Input: part model. Units: mm. Frame: model coordinates. Face numbers are marked on the shaded views. A direction names the side the tool comes from. Coordinates: 2 decimals unless noted, no trailing zeros. Order: outer loops, then holes, each group sorted by start corner. A loop starts at its lowest first (then second) coordinate and runs counter-clockwise, first axis right, second up.
from build123d import *

# Parameters (mm, degrees)
F0_R     = 1.27
F1_DEPTH = 13.096875
F2_W     = 19.84375
F2_H     = 11.90625
F3_DEPTH = 30.1635
F5_DEPTH = 26.19475
F7_R     = 4.7625
F8_DEPTH = 22.226


with BuildPart() as f1:
    # F0 (on Top) → F1 (new body, symmetric)
    with BuildSketch(Plane.XY):
        Polygon((-15.08125, 0), (0, 0), (15.08125, 0), (15.08125, 26.19375), (7.14375, 26.19375), (7.14375, 7.9375), (0, 7.9375), (-7.14375, 7.9375), (-7.14375, 26.19375), (-15.08125, 26.19375), align=None)
        with Locations((-11.1125, 22.225)):
            Circle(F0_R, mode=Mode.SUBTRACT)
        with Locations((11.1125, 22.225)):
            Circle(F0_R, mode=Mode.SUBTRACT)
    extrude(amount=F1_DEPTH, both=True)

    # F2 (on face) → F3 (cut, through all)
    with BuildSketch(Plane(origin=(-15.08125, 0, 0), x_dir=(0, -1, 0), z_dir=(-1, 0, 0))):
        with Locations((-16.271875, 7.14375)):
            Rectangle(F2_W, F2_H)
    extrude(amount=-F3_DEPTH, mode=Mode.SUBTRACT)

    # F4 (on face) → F5 (cut, through all)
    with BuildSketch(Plane.XZ):
        with BuildLine():
            ThreePointArc((-2.54, 13.096875), (0, 10.556875), (2.54, 13.096875))
            Line((2.54, 13.096875), (-2.54, 13.096875))
        make_face()
    extrude(amount=-F5_DEPTH, mode=Mode.SUBTRACT)

    # F7 (on offset) → F8 (cut, through all)
    with BuildSketch(Plane(origin=(0, 3.96875, 0), x_dir=(-1, 0, 0), z_dir=(0, 1, 0))):
        with Locations((0, 13.096875)):
            Circle(F7_R)
    extrude(amount=F8_DEPTH, mode=Mode.SUBTRACT)


solid = f1.part
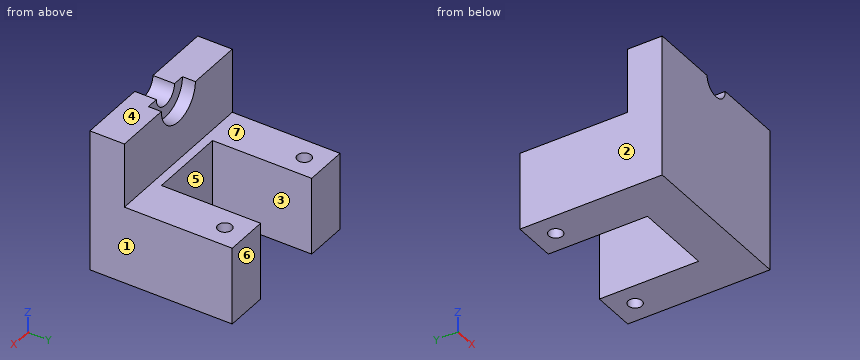
Item 1: Ray query, probe 1 along X at (y, z) = (22.25, -1); probe 2 along X at (y, z) = (14.25, -6); probe 3 along X at (y, z) = (22.75, -11.5). Return the intervals inside material, ascending.
Response values:
probe 1: x = -15.08 to -12.38, -9.84 to -7.14, 7.14 to 9.84, 12.38 to 15.08
probe 2: x = -15.08 to -7.14, 7.14 to 15.08
probe 3: x = -15.08 to -12.27, -9.96 to -7.14, 7.14 to 9.96, 12.27 to 15.08
Item 2: Access query for the marked faces 5, 6 and 7. Directions: +Z, -Z, +X, -X, +Y, -Y. A direction counts if a zero-diameter tool reaches every point of the face in a straight line with its end or side. Return the directions, or none.
Response values:
face 5: +Z, -Z, +Y
face 6: +Z, -Z, +X, -X, +Y
face 7: +Z, +X, -X, +Y
Item 3: Cut plane C-C on z = -4. Return loops of the section in (x, y) (1 decimal).
Response values:
outline: (-15.1, 0) - (15.1, 0) - (15.1, 26.2) - (7.1, 26.2) - (7.1, 7.9) - (-7.1, 7.9) - (-7.1, 26.2) - (-15.1, 26.2) - close; hole circle Ø2.5 at (-11.1, 22.2); hole circle Ø2.5 at (11.1, 22.2)
Item 4: Cut plane A-A on y = 8.75. Return loops of the section in (x, z).
Response values:
outline: (-15.08, -13.1) - (-7.14, -13.1) - (-7.14, 1.19) - (-15.08, 1.19) - close; (7.14, -13.1) - (15.08, -13.1) - (15.08, 1.19) - (7.14, 1.19) - close
Item 5: Pin query (flat end, axial travel): pin 1 Ø10 at (x, y) = (4.5, 20) entering from +Z; pin 2 Ø3 at (x, z) = (-9, 8.5) entering from +Y; pin 3 Ø2.5 at (x, z) = (-1.5, 11.5) entering from +Y. Return the tip coordinate at first contact, or that it passes through.
Response values:
pin 1: stops at z = 1.19
pin 2: stops at y = 6.35
pin 3: stops at y = 3.97
Item 6: Draft query along X for the marked faces 1, 2, 3 and 4. Return one class per face: pulls with the +X half, pulls with the -X half, needs draft (parallel to the pull), parting line crosses it, or undercut.
Response values:
face 1: pulls with the +X half
face 2: pulls with the -X half
face 3: undercut
face 4: needs draft
Item 7: Cut plane B-B on x = -11. Return loops of the section in (y, z), then the cut area to 3 significant figures.
Response values:
outline: (0, -13.1) - (20.96, -13.1) - (20.96, 1.19) - (6.35, 1.19) - (6.35, 13.1) - (0, 13.1) - close; (23.49, -13.1) - (26.19, -13.1) - (26.19, 1.19) - (23.49, 1.19) - close
area: 414 mm2
Item 8: Cut plane D-D on x = 0. Return loops of the section in (y, z), then the cut area to 3 significant figures.
Response values:
outline: (0, -13.1) - (7.94, -13.1) - (7.94, 1.19) - (6.35, 1.19) - (6.35, 8.33) - (3.97, 8.33) - (3.97, 10.56) - (0, 10.56) - close
area: 168 mm2
